```python
from build123d import *

# Parameters (mm, degrees)
SKETCH1_R                       = 48.5
SKETCH1_R_2                     = 1.5
BOSS_EXTRUDE1_DEPTH             = 4
SKETCH6_R                       = 3.75
CUT_EXTRUDE15_DEPTH             = 1.5
BOSS_EXTRUDE3_START             = 4
SKETCH5_R                       = 9
BOSS_EXTRUDE3_DEPTH             = 14
CUT_EXTRUDE16_START             = 6
SKETCH9_R                       = 1.3
CUT_EXTRUDE16_DEPTH             = 91.444646155
BOSS_EXTRUDE4_DEPTH             = 9
BOSS_EXTRUDE4_DIRECTION_2_REACH = 108.638
CUT_EXTRUDE17_DEPTH             = 101.75311462
CUT_EXTRUDE17_DEPTH_BACK        = 101.75311462
FILLET2_R                       = 10
FILLET3_R                       = 2


with BuildPart() as part:
    # Sketch1 → Boss-Extrude1 (new body)
    with BuildSketch(Plane(origin=(0, 0, 0), x_dir=(1, 0, 0), z_dir=(0, 1, 0))):
        with Locations(Location((0, 0, 0), (0, 0, 270))):
            Circle(SKETCH1_R)
        with Locations(Location((0, 7.25, 0), (0, 0, 270))):
            Circle(SKETCH1_R_2, mode=Mode.SUBTRACT)
        with Locations(Location((0, -7.25, 0), (0, 0, 270))):
            Circle(SKETCH1_R_2, mode=Mode.SUBTRACT)
    extrude(amount=BOSS_EXTRUDE1_DEPTH)

    # Sketch6 → Cut-Extrude15 (cut)
    with BuildSketch(Plane.XZ):
        with Locations(Location((0, 0, 0), (0, 0, 270))):
            Circle(SKETCH6_R)
    extrude(amount=-CUT_EXTRUDE15_DEPTH, mode=Mode.SUBTRACT)

    # Sketch5 → Boss-Extrude3 (add)
    with BuildSketch(Plane(origin=(0, 0, 0), x_dir=(0, 0, -1), z_dir=(1, 0, 0)).offset(BOSS_EXTRUDE3_START)):
        with BuildLine():
            Line((-30.34, 4), (30.34, 4))
            Line((30.34, 4), (30.34, 11.64))
            ThreePointArc((30.34, 11.64), (31.352340729, 17.057138369), (34.252718415, 21.743078098))
            ThreePointArc((34.252718415, 21.743078098), (30.606439261, 62.158587297), (-9.338476496, 55.009290775))
            Line((-9.338476496, 55.009290775), (-24.869934587, 30.494686245))
            ThreePointArc((-24.869934587, 30.494686245), (-28.94485921, 21.456068574), (-30.34, 11.64))
            Line((-30.34, 11.64), (-30.34, 4))
        make_face()
        with Locations((13.91, 40.28)):
            Circle(SKETCH5_R, mode=Mode.SUBTRACT)
    extrude(amount=BOSS_EXTRUDE3_DEPTH)

    # Sketch9 → Cut-Extrude16 (cut, through all)
    with BuildSketch(Plane(origin=(0, 0, 0), x_dir=(0, 0, -1), z_dir=(1, 0, 0)).offset(CUT_EXTRUDE16_START)):
        with Locations(Location((26.926504294, 47.525999231, 0), (0, 0, 180))):
            Circle(SKETCH9_R)
        with Locations(Location((19.855436483, 54.597067043, 0), (0, 0, 180))):
            Circle(SKETCH9_R)
        with Locations(Location((-7.014621202, 13.584873734, 0), (0, 0, 180))):
            Circle(SKETCH9_R)
        with Locations(Location((-14.085689014, 20.655941546, 0), (0, 0, 180))):
            Circle(SKETCH9_R)
        Polygon((0.41, 11.11), (29.401378029, 40.101378029), (12.43081528, 57.071940777), (-16.560562748, 28.080562748), align=None)
    extrude(amount=CUT_EXTRUDE16_DEPTH, mode=Mode.SUBTRACT)

    # Sketch10 → Boss-Extrude4 (add)
    with BuildSketch(Plane(origin=(18, 0, 0), x_dir=(0, 0, -1), z_dir=(1, 0, 0))):
        with BuildLine():
            Line((36.34, 4), (36.34, 11.64))
            ThreePointArc((36.34, 11.64), (36.947404437, 14.890283021), (38.687631049, 17.701846859))
            ThreePointArc((38.687631049, 17.701846859), (34.246427187, 66.928334449), (-14.406872962, 58.22042099))
            Line((-14.406872962, 58.22042099), (-29.938331054, 33.705816459))
            ThreePointArc((-29.938331054, 33.705816459), (-34.707253625, 23.127837278), (-36.34, 11.64))
            Line((-36.34, 11.64), (-36.34, 4))
            Line((-36.34, 4), (-27.34, 4))
            ThreePointArc((-27.34, 4), (-21.853757974, 30.744943155), (-9.338476496, 55.009290775))
            ThreePointArc((-9.338476496, 55.009290775), (30.606439261, 62.158587297), (34.252718415, 21.743078098))
            ThreePointArc((34.252718415, 21.743078098), (31.352340729, 17.057138369), (30.34, 11.64))
            Line((30.34, 11.64), (30.34, 4))
            Line((30.34, 4), (36.34, 4))
        make_face()
    extrude(amount=BOSS_EXTRUDE4_DEPTH)

    # Boss-Extrude4 direction 2: up to this face of the body (flat: up to its plane)
    boss_extrude4_direction_2_end = Plane(part.part.faces().sort_by_distance((4, 32.000082857, -6.789790598))[0])
    # Sketch10 → Boss-Extrude4 direction 2 (add, up to the picked face)
    with BuildSketch(Plane(origin=(18, 0, 0), x_dir=(0, 0, -1), z_dir=(1, 0, 0)), mode=Mode.PRIVATE) as boss_extrude4_direction_2_sk1:
        with BuildLine():
            Line((36.34, 4), (36.34, 11.64))
            ThreePointArc((36.34, 11.64), (36.947404437, 14.890283021), (38.687631049, 17.701846859))
            ThreePointArc((38.687631049, 17.701846859), (34.246427187, 66.928334449), (-14.406872962, 58.22042099))
            Line((-14.406872962, 58.22042099), (-29.938331054, 33.705816459))
            ThreePointArc((-29.938331054, 33.705816459), (-34.707253625, 23.127837278), (-36.34, 11.64))
            Line((-36.34, 11.64), (-36.34, 4))
            Line((-36.34, 4), (-27.34, 4))
            ThreePointArc((-27.34, 4), (-21.853757974, 30.744943155), (-9.338476496, 55.009290775))
            ThreePointArc((-9.338476496, 55.009290775), (30.606439261, 62.158587297), (34.252718415, 21.743078098))
            ThreePointArc((34.252718415, 21.743078098), (31.352340729, 17.057138369), (30.34, 11.64))
            Line((30.34, 11.64), (30.34, 4))
            Line((30.34, 4), (36.34, 4))
        make_face()
    boss_extrude4_direction_2_tool1 = split(extrude(boss_extrude4_direction_2_sk1.sketch, amount=-BOSS_EXTRUDE4_DIRECTION_2_REACH, mode=Mode.PRIVATE), bisect_by=boss_extrude4_direction_2_end, keep=Keep.BOTH, mode=Mode.PRIVATE)
    add(boss_extrude4_direction_2_tool1.solids().sort_by(Axis((18, 63.025419, -31.267953), (-1, 0, 0)))[0])

    # Sketch11 → Cut-Extrude17 (cut, two sides: drawn at the far end of the back side and taken through both)
    with BuildSketch(Plane.XY.offset(-CUT_EXTRUDE17_DEPTH_BACK)):
        with BuildLine():
            Line((27, 73.801694463), (21, 73.801694463))
            ThreePointArc((21, 73.801694463), (22.52665425, 38.804454133), (26.5, 4))
            Line((26.5, 4), (27, 4))
            Line((27, 4), (27, 73.801694463))
        make_face()
    extrude(amount=CUT_EXTRUDE17_DEPTH + CUT_EXTRUDE17_DEPTH_BACK, mode=Mode.SUBTRACT)

    # Fillet2
    # the kernel refuses this fillet: 10 mm, written as the material it takes off along each edge
    with BuildSketch(Plane(origin=(4, 40.28, -13.91), x_dir=(0, -0.6735385398377843, -0.7391521056948872), z_dir=(0, -0.7391521056948872, 0.6735385398377843))) as fillet2_piece_1:
        with BuildLine():
            CenterArc((33.521694463 - FILLET2_R, FILLET2_R), FILLET2_R, 270, 90)
            Line((33.521694463, FILLET2_R), (33.521694463, 0))
            Line((33.521694463, 0), (33.521694463 - FILLET2_R, 0))
        make_face()
    revolve(axis=Axis((4, 40.28, -13.91), (1, 0, 0)), revolution_arc=189.984074965, mode=Mode.SUBTRACT)
    with BuildSketch(Plane(origin=(4, 58.22042099, 14.406872962), x_dir=(0, -0.5351883691335427, -0.8447327444489049), z_dir=(0, -0.8447327444489049, 0.5351883691335426))) as fillet2_piece_2:
        with BuildLine():
            CenterArc((FILLET2_R, FILLET2_R), FILLET2_R, 180, 90)
            Line((0, FILLET2_R), (0, 0))
            Line((0, 0), (FILLET2_R, 0))
        make_face()
    extrude(amount=29.020544891, mode=Mode.SUBTRACT)
    with BuildSketch(Plane(origin=(4, 11.64, -4.89), x_dir=(0, 0.5351883691335412, 0.8447327444489058), z_dir=(0, 0.8447327444489058, -0.5351883691335412))) as fillet2_piece_3:
        with BuildLine():
            CenterArc((41.23 - FILLET2_R, FILLET2_R), FILLET2_R, 270, 90)
            Line((41.23, FILLET2_R), (41.23, 0))
            Line((41.23, 0), (41.23 - FILLET2_R, 0))
        make_face()
    revolve(axis=Axis((4, 11.64, -4.89), (1, 0, 0)), revolution_arc=32.356687045, mode=Mode.SUBTRACT)
    with BuildSketch(Plane(origin=(4, 11.64, 36.34), x_dir=(0, 0, -1), z_dir=(0, -1, 0)), Plane(origin=(4, 4, -36.34), x_dir=(0, 0, 1), z_dir=(0, 1, 0))) as fillet2_piece_4:
        with BuildLine():
            CenterArc((FILLET2_R, FILLET2_R), FILLET2_R, 180, 90)
            Line((0, FILLET2_R), (0, 0))
            Line((0, 0), (FILLET2_R, 0))
        make_face()
    extrude(amount=7.64, mode=Mode.SUBTRACT)
    with BuildSketch(Plane(origin=(4, 11.64, -45.34), x_dir=(0, 0.6735385398377856, 0.739152105694886), z_dir=(0, 0.739152105694886, -0.6735385398377856))) as fillet2_piece_5:
        with BuildLine():
            CenterArc((9 + FILLET2_R, FILLET2_R), FILLET2_R, 180, 90)
            Line((9, FILLET2_R), (9, 0))
            Line((9, 0), (9 + FILLET2_R, 0))
        make_face()
    revolve(axis=Axis((4, 11.64, -45.34), (1, 0, 0)), revolution_arc=42.340762009, mode=Mode.SUBTRACT)

    # Fillet3
    fillet3_edges = [part.edges().sort_by_distance(p)[0] for p in [
        (20.25, 4, -36.34),
        (20.25, 4, 36.34),
        (6.928932188, 4, 33.411067812),
        (4, 4, 0),
        (6.928932188, 4, -33.411067812),
    ]]
    fillet(fillet3_edges, radius=FILLET3_R)
    fillet3_2_edges = [part.edges().sort_by_distance(p)[0] for p in [
        (26.5, 4, -33.34),
    ]]
    fillet(fillet3_2_edges, radius=FILLET3_R)
    fillet3_3_edges = [part.edges().sort_by_distance(p)[0] for p in [
        (26.5, 4, 31.84),
    ]]
    fillet(fillet3_3_edges, radius=FILLET3_R)


solid = part.part
```
Could you check a few things on this model? Use its own coordinates, in mm. A direction names the side the tool comes from. Coordinates: 2 decimals unless noted, no trailing zeros. Loops run counter-clockwise (first coordinate to the right, second up) from the corner with the lowest first, then second, coordinate; pieces in that order, holes last. Notation, with made-up numbers: M 53,-23 L 77,-23 A7 cw 77,-18 Z; hole C 57.5,1 d4. An arc over 180 degrees is marked long. Put each result on its own line as item: value. Start each with the question number.
(1) Will these pins go through, and if not, where does the flat tip stop? P1, Ø4.5, axis at x = 19.5, y = 7.5, coming from the -Z side; P2, Ø6, axis at x = 24.5, y = 8.5, coming from the +Z side; P3, Ø1, axis at y = 51, z = -25.5, coming from the -X side.
(2) For faces 1 (the face through (7.01, 8.86, 33.49)), 2 (the face through (4, 28, -5)), 3 (the face through (18.21, 66.45, -34.86)), 4 (the face through (0.07, 1.97, 5.75)), 5 (the face through (11.9, 48.5, -21)), which set-ups out of +Z, -Z, +X, -X, +Y, -Y let a thin tool reach every point of the face, with its end or its side?
(3) Suppose I cut it at B-B on z = -7.25. Count the separate pieces of the cut face and the enclosed holes in it, then the cut area to 3 significant figures.
(4) Suppose I cut it at A-A on x = 0. Please give me the cut outline in (y, z), then the cut area to 3 significant figures.
(5) Thinking about a two-plate mould opening in X: for faces 6 (the face through (0, 1.5, 0)), 7 (the face through (6, 14, 7)), 8 (the face through (7.01, 44.61, 19.66)), 9 (the face through (18.54, 46.135, 22.064)), which applies, pulls with the +X half, pulls with the -X half, needs draft (parallel to the pull), parting line crosses it, or undercut?
(6) I need wall thicknesses on line 1 (Y direction, x = 22.75, z = -13.91); line 2 (X direction, y = 2.2, z = 7.25); line 3 (X direction, y = 15, z = 5). Which ranges of each line are inside material? Lowest first, please. Write a range as from..to.
(7) Suppose I cut it at C-C on x = -16. Please give me the cut outline in (y, z), then the cut area to 3 significant figures.
Solutions:
1. P1: stops at z = -36.49
1. P2: stops at z = 36.4
1. P3: stops at x = 4
2. face 1: +Z, -X, +Y
2. face 2: +Z, -Z, -X, +Y
2. face 3: +X, -X
2. face 4: +Y, -Y
2. face 5: +X
3. separate pieces: 3
3. enclosed holes: 0
3. area: 906 mm2
4. outline: M 0,-48.5 L 4,-48.5 L 4,-8.75 L 0,-8.75 Z; M 0,-5.75 L 4,-5.75 L 4,5.75 L 0,5.75 L 0,3.75 L 1.5,3.75 L 1.5,-3.75 L 0,-3.75 Z; M 0,8.75 L 4,8.75 L 4,48.5 L 0,48.5 Z
4. area: 353 mm2
5. face 6: undercut
5. face 7: pulls with the +X half
5. face 8: pulls with the -X half
5. face 9: needs draft
6. line 1: y = 0..4
6. line 2: x = -47.96..-1.5, 1.5..47.96
6. line 3: x = 4..18
7. outline: M 0,-45.78 L 4,-45.78 L 4,45.78 L 0,45.78 Z
7. area: 366 mm2
